Build history of the part. All positions in model axes, mm. Face numbers are marked on the shaded views. Coordinates: 2 decimals unless noted, no trailing zeros. Loops run counter-clockwise (first coordinate to the right, second up) from the corner with the lowest first, then second, coordinate; pieces in that order, holes last.
Item 1: Cut at B-B (x = -1.5). List the corners of the cut face in (y, z).
Item 2: Mould opens along X. For the marked faces 1, 2 and 3 say: released by +X, released by -X, zero draft, split by the parting line, or undercut.
Item 3: Cut at A-A (z = 57.5). List the corners of the cut face in (x, y).
Item 4: Flat gauge pins, fed straight in: pin 1 (1.5 mm diameter, centred on x = 6.5, y = -7, fed in from -Z); pin 2 (1.2 mm diameter, centred on x = 1.5, y = -1, fed in from +Z); pin 3 (1.5 mm diameter, centred on y = -3, z = 20.5, fed in from -X). Where does each tip first touch, or does it go through?
Item 5: Cut at D-D (z = 44). List the corners of the cut face in (x, y), and give its area (3 significant figures).
Item 6: Cut at C-C (y = -5). Count the separate pieces of the cut face and the enclosed holes in it, and give its area (3 significant figures).
Item 7: Drill centre lines: line 1 along Z through (x, y) = (0, -9.05); line 2 along Z through (x, y) = (0, -8.25); line 3 along Z through (x, y) = (-1.5, -1.75). Where is each one in solid material? Low to high.
Autodesk Inventor part; units mm, degrees
ref_plane "Work Plane3" through (0, 0, 79.75) normal (0, 0, -1) x (-1, 0, 0)
ref_plane "YZ Plane" through (0, 0, 0) normal (1, 0, 0) x (0, 1, 0)
ref_plane "XZ Plane" through (0, 0, 0) normal (0, 1, 0) x (-1, 0, 0)
sketch "Sketch1" plane through (0, 0, 0) normal (0, 1, 0) x (-1, 0, 0)
  circle A0 centre (-0.0087, 99.7911) radius 10
  circle A1 centre (-0.0022, 9.7911) radius 15
  line L0 (9.9759, 100.3474) -> (14.9746, 10.6255)
  line L1 (-9.9933, 100.346) -> (-14.9791, 10.6234)
  point P0 (0, 0)
  dimension "d0" = 20
  dimension "d1" = 30
  dimension "d2" = 90
extrude "Extrusion1" add sketch "Sketch1" against normal blind 10
sketch "Sketch2" plane through (0, 0, 0) normal (0, 1, 0) x (1, 0, 0)
  circle A0 centre (0, -99.8683) radius 3.75
  circle A1 centre (0, -83.8683) radius 2.75
  line L0 (2.7446, -83.6964) -> (3.7427, -99.6339)
  line L1 (-3.7427, -99.6339) -> (-2.7446, -83.6964)
  point P0 (0, 0)
  dimension "d7" = 7.5
  dimension "d8" = 5.5
  dimension "d9" = 16
extrude "Extrusion2" cut sketch "Sketch2" against normal blind 8.5
sketch "Sketch3" plane through (0, -8.5, 0) normal (0, 1, 0) x (1, 0, 0)
  arc A0 (-3.7427, -99.6339) -> (3.7427, -99.6339) centre (0, -99.8683) ccw
  circle A1 centre (0, -99.8683) radius 3.65
  point P0 (0, 0)
  dimension "d12" = 7.3
extrude "Extrusion3" cut sketch "Sketch3" against normal blind 8.5
sketch "Sketch4" plane through (0, 0, 0) normal (0, 1, 0) x (1, 0, 0)
  arc A0 (14.9791, -10.6234) -> (-14.9746, -10.6255) centre (0.0022, -9.7911) ccw
  circle A1 centre (0.0022, -9.7911) radius 5.25
  point P0 (0, 0)
  dimension "d15" = 10.5
extrude "Extrusion4" cut sketch "Sketch4" against normal blind 11
sketch "Sketch6" plane through (0, 0, 0) normal (0, 0, 1) x (1, 0, 0)
  line L0 (-10.7414, -1.5061) -> (11.4058, -1.5061)
  line L1 (11.4058, -1.5061) -> (11.4058, -8.375)
  line L2 (11.4058, -8.375) -> (-10.7414, -8.375)
  line L3 (-10.7414, -8.375) -> (-10.7414, -1.5061)
  point P0 (0, 0)
extrude "Extrusion6" add sketch "Sketch6" along normal blind 1
ref_plane "Work Plane3" through (0, 0, 79.75) normal (0, 0, -1) x (-1, 0, 0)
sketch "Sketch7" plane through (0, 0, 79.75) normal (0, 0, -1) x (-1, 0, 0)
  line L0 (5.25, -1.5083) -> (-5.25, -1.5083)
  line L1 (-5.25, -1.5083) -> (-5.25, -8.8083)
  line L2 (-5.25, -8.8083) -> (5.25, -8.8083)
  line L3 (5.25, -8.8083) -> (5.25, -1.5083)
  line L4 (5.25, -1.5083) -> (-5.25, -8.8083) construction
  line L5 (-5.25, -1.5083) -> (5.25, -8.8083) construction
  point P0 (0, 0)
  point P1 (0, -5.1583)
  dimension "d23" = 10.5
  dimension "d24" = 7.3
extrude "Extrusion7" cut sketch "Sketch7" along normal blind 62.25
sketch "Sketch8" plane through (0, 0, 0) normal (0, 1, 0) x (1, 0, 0)
  line L0 (-5, -79.6503) -> (5, -79.6503)
  line L1 (5, -79.6503) -> (5, -74.6503)
  line L2 (5, -74.6503) -> (-5, -74.6503)
  line L3 (-5, -74.6503) -> (-5, -79.6503)
  line L4 (-5, -79.6503) -> (5, -74.6503) construction
  line L5 (5, -79.6503) -> (-5, -74.6503) construction
  point P0 (0, 0)
  point P1 (0, -77.1503)
  dimension "d27" = 10
  dimension "d28" = 5
extrude "Extrusion8" cut sketch "Sketch8" against normal blind 8.5
sketch "Sketch9" plane through (-14.9746, -10, 10.6255) normal (-0.9985, 0, 0.0556) x (0.0556, 0, 0.9985)
  line L0 (16.1756, 2.6337) -> (6.1756, 2.6337)
  line L1 (6.1756, 2.6337) -> (6.1756, 7.6337)
  line L2 (6.1756, 7.6337) -> (16.1756, 7.6337)
  line L3 (16.1756, 7.6337) -> (16.1756, 2.6337)
  line L4 (16.1756, 2.6337) -> (6.1756, 7.6337) construction
  line L5 (6.1756, 2.6337) -> (16.1756, 7.6337) construction
  point P0 (-9.7761, 10)
  point P1 (11.1756, 5.1337)
  dimension "d31" = 10
  dimension "d32" = 5
extrude "Extrusion9" cut sketch "Sketch9" against normal blind 20.5
properties part number "Brazo_3DPrint"
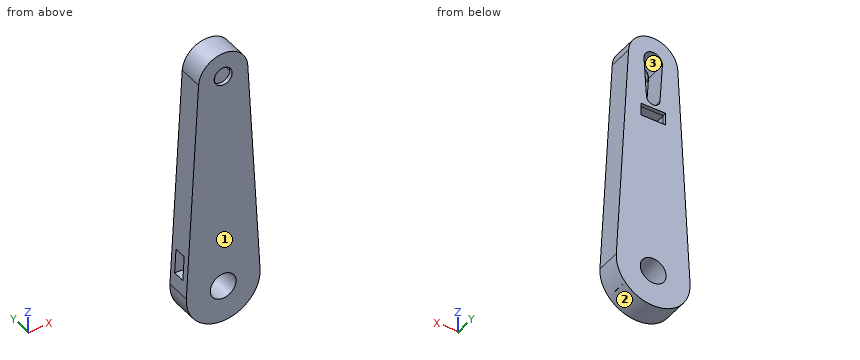
Filled sheet:
1. outline: (-10, -5.13) - (0, -5.13) - (0, 4.76) - (-10, 4.76) - close; (-10, 14.82) - (0, 14.82) - (0, 74.65) - (-1.51, 74.65) - (-1.51, 17.5) - (-2.37, 17.5) - (-2.37, 16.06) - (-7.37, 16.06) - (-7.37, 17.5) - (-8.81, 17.5) - (-8.81, 79.75) - (-1.51, 79.75) - (-1.51, 79.65) - (0, 79.65) - (0, 81.56) - (-8.5, 81.56) - (-8.5, 96.54) - (-10, 96.54) - close; (-10, 103.2) - (-8.5, 103.2) - (-8.5, 103.31) - (0, 103.31) - (0, 109.68) - (-10, 109.68) - close
2. face 1: zero draft
2. face 2: split by the parting line
2. face 3: undercut
3. outline: (-12.36, -10) - (12.37, -10) - (12.37, 0) - (-12.36, 0) - close; hole (-5.25, -8.81) - (5.25, -8.81) - (5.25, -1.51) - (-5.25, -1.51) - close
4. pin 1: stops at z = -4.06
4. pin 2: stops at z = 109.75
4. pin 3: stops at x = -14.45
5. outline: (-13.12, -10) - (13.12, -10) - (13.12, 0) - (-13.12, 0) - close; hole (-5.25, -8.81) - (5.25, -8.81) - (5.25, -1.51) - (-5.25, -1.51) - close
5. area: 186 mm2
6. separate pieces: 1
6. enclosed holes: 2
6. area: 1,770 mm2
7. line 1: z = -5.21 to 4.54, 15.04 to 96.22, 103.52 to 109.79
7. line 2: z = -5.21 to 4.54, 15.04 to 17.5, 79.75 to 81.12, 103.62 to 109.79
7. line 3: z = -5.13 to 4.76, 14.82 to 17.5, 79.75 to 81.56, 103.31 to 109.68
